Read the model definition and answer for the solid it produces. Units are mm, in the model's axes. Face numbers are marked on the shaded views. Coordinates: 2 decimals unless noted, no trailing zeros. Loops run counter-clockwise (first coordinate to the right, second up) from the corner with the lowest first, then second, coordinate; pieces in that order, holes last. Notation, with made-up numbers: (48, 45.25) - (107, 45.25) arc R29 cw to (107, 75.25) - close; hole circle Ø4 at (-20.5, -38). An arc over 180 degrees is marked (long way). Use one line per item in the form item = value.
from build123d import *

# Parameters (mm, degrees)
SKETCH1_W           = 90
SKETCH1_H           = 170
BOSS_EXTRUDE1_DEPTH = 7.5
SKETCH2_W           = 86
SKETCH2_H           = 166
BOSS_EXTRUDE2_DEPTH = 7.5
SKETCH5_W           = 72
SKETCH5_H           = 152
CUT_EXTRUDE1_DEPTH  = 7.5


with BuildPart() as part:
    # Sketch1 → Boss-Extrude1 (new body)
    with BuildSketch(Plane(origin=(0, 0, 0), x_dir=(1, 0, 0), z_dir=(0, 1, 0))):
        Rectangle(SKETCH1_W, SKETCH1_H)
    extrude(amount=BOSS_EXTRUDE1_DEPTH)

    # Sketch2 → Boss-Extrude2 (add)
    with BuildSketch(Plane.XZ):
        Rectangle(SKETCH2_W, SKETCH2_H)
    extrude(amount=BOSS_EXTRUDE2_DEPTH)

    # Sketch5 → Cut-Extrude1 (cut)
    with BuildSketch(Plane.XZ.offset(7.5)):
        Rectangle(SKETCH5_W, SKETCH5_H)
    extrude(amount=-CUT_EXTRUDE1_DEPTH, mode=Mode.SUBTRACT)


solid = part.part
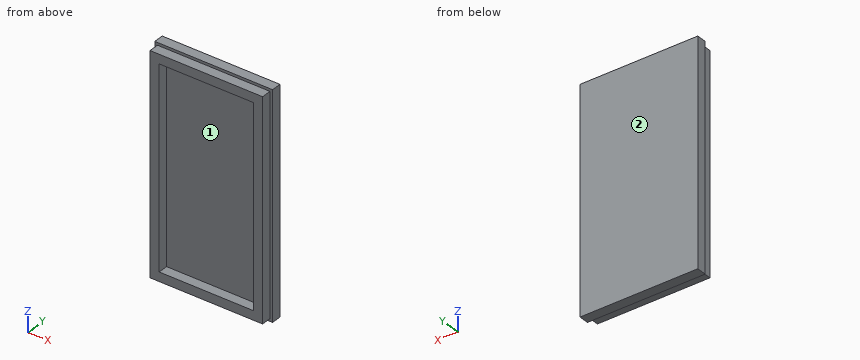
Item 1: For a pull along X with two mould halves and no side action, classify the marked faces 1 and 2 as +X half, -X half, draft (parallel to the pull), parting line (faces both ways), or undercut.
Results below:
face_1 = undercut
face_2 = draft
Item 2: The part is cut by section C-C on z = -59.5. Give the vertices of the cut face in (x, y).
Results below:
outline = (-45, 0) - (-43, 0) - (-43, -7.5) - (-36, -7.5) - (-36, 0) - (36, 0) - (36, -7.5) - (43, -7.5) - (43, 0) - (45, 0) - (45, 7.5) - (-45, 7.5) - close
Item 3: Each of these flat-tipped pins is pushed along its axis until it touches: P1, Ø8, axis at x = 30, z = -25, coming from the -Y side; P2, Ø3, axis at x = 29, y = -5.5, coming from the +Z side; P3, Ø8, axis at x = -12, y = -3, coming from the -Z side; P4, Ø2, axis at y = -5, z = 32.5, coming from the -X side. Where does it stop, or does it pass through?
Results below:
P1 = 0
P2 = 83
P3 = -85
P4 = -43
Item 4: The part is cut by section B-B on x = -10. Give the vertices of the cut face in (y, z).
Results below:
outline = (-7.5, -83) - (0, -83) - (0, -85) - (7.5, -85) - (7.5, 85) - (0, 85) - (0, 83) - (-7.5, 83) - (-7.5, 76) - (0, 76) - (0, -76) - (-7.5, -76) - close
Item 5: The part is cut by section A-A on y = -2. Give the vertices of the cut face in (x, z), plus the area to 3 significant figures.
Results below:
outline = (-43, -83) - (43, -83) - (43, 83) - (-43, 83) - close; hole (-36, -76) - (36, -76) - (36, 76) - (-36, 76) - close
area = 3,330 mm²
Item 6: Find the intervals of material crossed by L1, parallel to X at y = -1.75, z = 66.5; L2, parallel to Y at x = -14, z = -21.5; L3, parallel to Z at x = 7, y = -3.75, in increasing order.
Results below:
L1 = -43 to -36, 36 to 43
L2 = 0 to 7.5
L3 = -83 to -76, 76 to 83
